Check sheet for the drawn part. Datum: minimum x, y, z corner. Units: mm. Give positions to 0.01 mm unless a question says otherwise; leave off trailing zeros. Loops run counter-clockwise (first coordinate to the right, second up) from the corner with the lowest first, then second, coordinate; pieces in that order, holes last. Notation, with made-up numbers: (-14, -24) - (-4, -24) arc R21 cw to (-4, -2) - close; hole circle Ø2 at (16, 41). An arc over 180 degrees is marked (long way). Use a Markdown table: item, result. Add a question column.
1. Cross-section at A-A on y = 7. Enter the section's corners in (x, z) (1 decimal).
2. Depth check by flat-ended pin: P1, Ø1.5, axis at x = 12, y = 89, coming from the +Z side (1 decimal); P2, Ø2, axis at y = 23, z = 10.5, coming from the +X side; P3, Ø1.3, axis at y = 18, z = 10, coming from the -X side. Enter the tip coordinate at first touch or a pass-through.
3. Material ranges on L1, parallel to Y at x = 7, z = 11.5; L2, parallel to X at y = 43, z = 3.5 (1 decimal); L3, parallel to X at y = 25, z = 4 (1 decimal), recorded low to high.
4. Cross-section at B-B on y = 93. Enter the section's corners in (x, z) (1 decimal).
5. Cross-section at C-C on x = 1.75. Enter the section's corners in (y, z).
6. Draft check along X on the marked faces 1, 2 and 3. Enter one of: pulls with the +X half, pulls with the -X half, needs draft (parallel to the pull), parting line crosses it, or undercut.
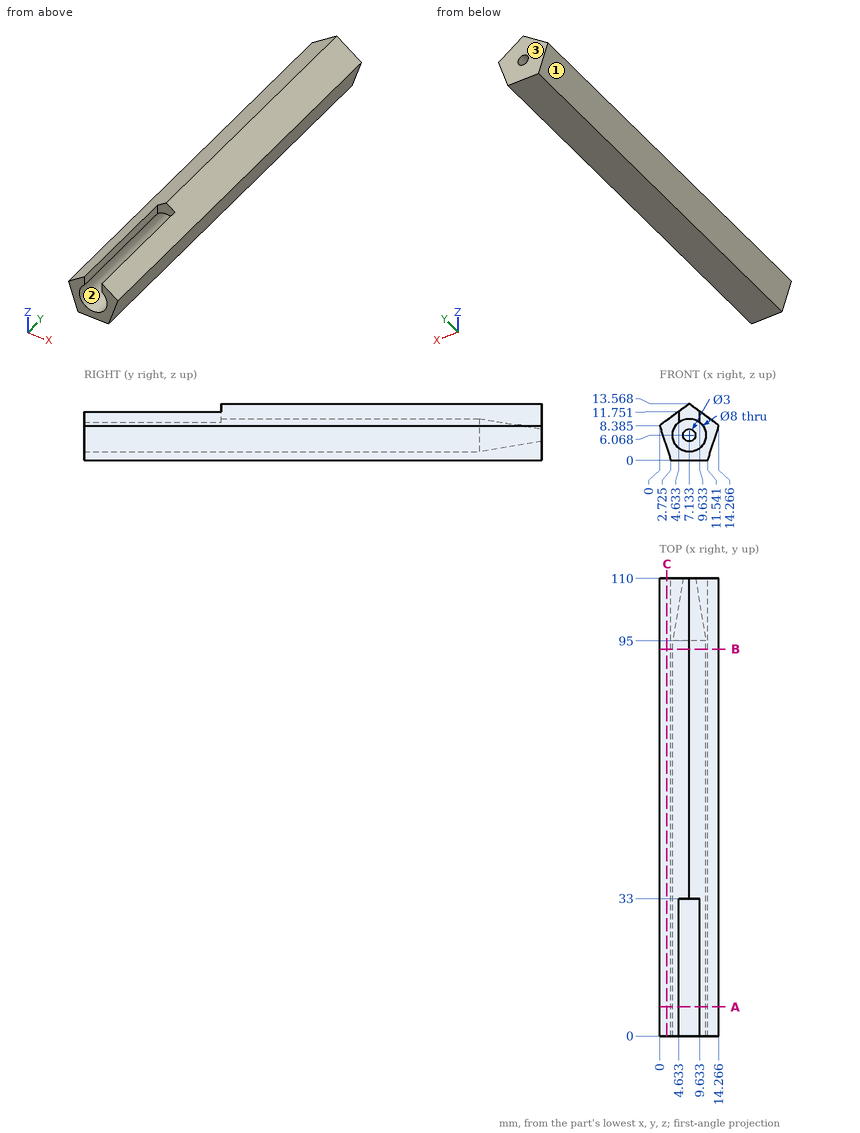
Values found:
| question | item | result |
|---|---|---|
| 1 | outline | (0, 8.4) - (2.7, 0) - (11.5, 0) - (14.3, 8.4) - (9.6, 11.8) - (9.6, 9.2) arc R4 cw (long way) to (4.6, 9.2) - (4.6, 11.8) - close |
| 2 | P1 | stops at z = 10.6 |
| 2 | P2 | stops at x = 12.73 |
| 2 | P3 | stops at x = 1.33 |
| 3 | L1 | y = 33 to 110 |
| 3 | L2 | x = 1.6 to 4.1, 10.2 to 12.7 |
| 3 | L3 | x = 1.4 to 3.7, 10.6 to 12.8 |
| 4 | outline | (0, 8.4) - (2.7, 0) - (11.5, 0) - (14.3, 8.4) - (7.1, 13.6) - close; hole circle Ø8 at (7.1, 6.1) |
| 5 | outline | (0, 3) - (110, 3) - (110, 9.66) - (0, 9.66) - close |
| 6 | face 1 | pulls with the -X half |
| 6 | face 2 | undercut |
| 6 | face 3 | needs draft |
